```python
from build123d import *

# Parameters (mm, degrees)
SKETCH_1_W          = 109
SKETCH_1_H          = 31
SKETCH_1_W_2        = 9.6
SKETCH_1_H_2        = 9.7
SKETCH_1_H_3        = 5.6
SKETCH_1_W_3        = 14.8
SKETCH_1_H_4        = 16
SKETCH_1_W_4        = 9.5
SKETCH_1_H_5        = 3.5
SKETCH_1_W_5        = 15.5
SKETCH_1_H_6        = 6
SKETCH_1_W_6        = 80
SKETCH_1_H_7        = 8
EXTRUDE_1_DEPTH     = 2
SKETCH_2_W          = 2.5
SKETCH_2_H          = 8
EXTRUDE_2_DEPTH     = 2
SKETCH_3_W          = 15
SKETCH_3_H          = 2.5
EXTRUDE_4_DEPTH     = 2
CUT_EXTRUDE_2_DEPTH = 2


with BuildPart() as part:
    # 草图1 → 凸台-拉伸1 (new body)
    with BuildSketch(Plane.XY):
        with Locations((43, 12.2)):
            Rectangle(SKETCH_1_W, SKETCH_1_H)
        Polygon((27.2, 3.55), (32.1, 3.55), (32.1, 0.55), (39, 0.55), (39, 3.55), (43.9, 3.55), (43.9, 13.55), (27.2, 13.55), align=None, mode=Mode.SUBTRACT)
        with Locations((4.8, 4.85)):
            Rectangle(SKETCH_1_W_2, SKETCH_1_H_2, mode=Mode.SUBTRACT)
        with Locations((18.5, 6.9)):
            Rectangle(SKETCH_1_W_2, SKETCH_1_H_3, mode=Mode.SUBTRACT)
        with Locations((54.7, 6.55)):
            Rectangle(SKETCH_1_W_3, SKETCH_1_H_4, mode=Mode.SUBTRACT)
        with Locations((76.35, 12.8)):
            Rectangle(SKETCH_1_W_4, SKETCH_1_H_5, mode=Mode.SUBTRACT)
        with Locations((76.35, 3.55)):
            Rectangle(SKETCH_1_W_5, SKETCH_1_H_6, mode=Mode.SUBTRACT)
        with Locations((43, 20.2)):
            Rectangle(SKETCH_1_W_6, SKETCH_1_H_7, mode=Mode.SUBTRACT)
    extrude(amount=EXTRUDE_1_DEPTH)

    # 草图2 → 凸台-拉伸2 (add)
    with BuildSketch(Plane.XY.offset(2)):
        with Locations((-12.75, 18.7)):
            Rectangle(SKETCH_2_W, SKETCH_2_H)
        with Locations((-12.75, 5.7)):
            Rectangle(SKETCH_2_W, SKETCH_2_H)
        with Locations((98.75, 5.7)):
            Rectangle(SKETCH_2_W, SKETCH_2_H)
        with Locations((98.75, 18.7)):
            Rectangle(SKETCH_2_W, SKETCH_2_H)
    extrude(amount=-EXTRUDE_2_DEPTH)

    # 草图3 → 凸台-拉伸4 (add)
    with BuildSketch(Plane.XY):
        with Locations((6, 28.95)):
            Rectangle(SKETCH_3_W, SKETCH_3_H)
        with Locations((43, 28.95)):
            Rectangle(SKETCH_3_W, SKETCH_3_H)
        with Locations((80, 28.95)):
            Rectangle(SKETCH_3_W, SKETCH_3_H)
        with Locations((80, -4.55)):
            Rectangle(SKETCH_3_W, SKETCH_3_H)
        with Locations((43, -4.55)):
            Rectangle(SKETCH_3_W, SKETCH_3_H)
        with Locations((6, -4.55)):
            Rectangle(SKETCH_3_W, SKETCH_3_H)
    extrude(amount=EXTRUDE_4_DEPTH)

    # 草图4 → 切除-拉伸2 (cut)
    with BuildSketch(Plane.XY):
        with BuildLine():
            Line((-3.5, 27.7), (-1.5, 27.7))
            ThreePointArc((-1.5, 27.7), (-2.5, 26.7), (-3.5, 27.7))
        make_face()
        with BuildLine():
            Line((15.5, 27.7), (13.5, 27.7))
            ThreePointArc((13.5, 27.7), (14.5, 26.7), (15.5, 27.7))
        make_face()
        with BuildLine():
            Line((33.5, 27.7), (35.5, 27.7))
            ThreePointArc((35.5, 27.7), (34.5, 26.7), (33.5, 27.7))
        make_face()
        with BuildLine():
            Line((52.5, 27.7), (50.5, 27.7))
            ThreePointArc((50.5, 27.7), (51.5, 26.7), (52.5, 27.7))
        make_face()
        with BuildLine():
            Line((70.5, 27.7), (72.5, 27.7))
            ThreePointArc((72.5, 27.7), (71.5, 26.7), (70.5, 27.7))
        make_face()
        with BuildLine():
            Line((89.5, 27.7), (87.5, 27.7))
            ThreePointArc((87.5, 27.7), (88.5, 26.7), (89.5, 27.7))
        make_face()
        with BuildLine():
            Line((89.5, -3.3), (87.5, -3.3))
            ThreePointArc((87.5, -3.3), (88.5, -2.3), (89.5, -3.3))
        make_face()
        with BuildLine():
            Line((70.5, -3.3), (72.5, -3.3))
            ThreePointArc((72.5, -3.3), (71.5, -2.3), (70.5, -3.3))
        make_face()
        with BuildLine():
            Line((52.5, -3.3), (50.5, -3.3))
            ThreePointArc((50.5, -3.3), (51.5, -2.3), (52.5, -3.3))
        make_face()
        with BuildLine():
            Line((33.5, -3.3), (35.5, -3.3))
            ThreePointArc((35.5, -3.3), (34.5, -2.3), (33.5, -3.3))
        make_face()
        with BuildLine():
            Line((15.5, -3.3), (13.5, -3.3))
            ThreePointArc((13.5, -3.3), (14.5, -2.3), (15.5, -3.3))
        make_face()
        with BuildLine():
            Line((-3.5, -3.3), (-1.5, -3.3))
            ThreePointArc((-1.5, -3.3), (-2.5, -2.3), (-3.5, -3.3))
        make_face()
    extrude(amount=CUT_EXTRUDE_2_DEPTH, mode=Mode.SUBTRACT)


solid = part.part
```
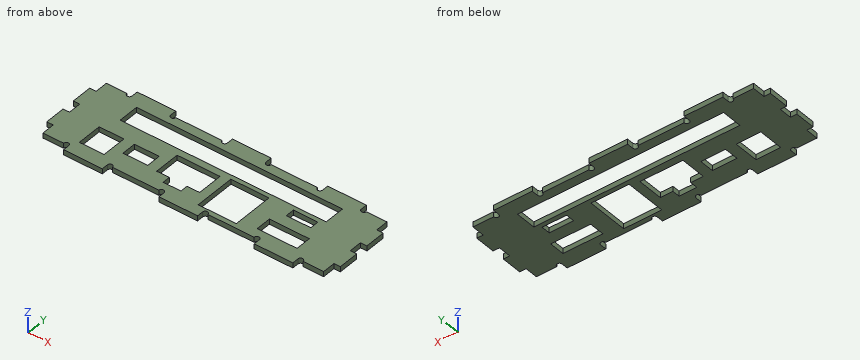
CAD build for the part. Positions are in the model's coordinates, mm. Round coordinates to 2 decimals unless told otherwise and drop trailing zeros. Write each loop counter-clockwise with the first axis right and the second up, starting at its lowest first coordinate (ties: lowest second). Pieces come first, ordered by that corner, then holes. Notation, with made-up numbers: (53, 48.25) - (90, 48.25) arc R23 cw to (90, 63.25) - close; hole circle Ø4 at (50.25, 52.25). An arc over 180 degrees is marked (long way). Write item = value, one per line. Start each with the question number.
Q1. Band-saw the part on A-A (x = 7). Give the cut face in (y, z), then the cut area to 3 significant figures.
Q2. Band-saw the part on B-B (y = 20). Give the cut face in (x, z), then the cut area to 3 significant figures.
Q3. Band-saw the part on D-D (z = 1.7). Count the separate pieces of the cut face and the enclosed holes in it, then the cut area to 3 significant figures.
Q4. Probe L1, parallel to Y at x = 81, z = 0.5; L2, parallel to Y at x = 8, z = 0.8; L3, parallel to X at y = 4, z = 0.5. List the from-to ranges inside material, lowest first. Write a range as from..to.
Q5. Band-saw the part on C-C (y = 8). Give the cut face in (x, z).
Q6. Drop flat-ended pins along their axis: pin 1 (0.6 mm diameter, centred on y = -1.5, z = 0.5, fed in from +X); pin 2 (0.6 mm diameter, centred on x = 25, z = 1, fed in from +Y). Give the stop position or say it passes through.
Answers below:
q1.outline = (-5.8, 0) - (0, 0) - (0, 2) - (-5.8, 2) - close; (9.7, 0) - (16.2, 0) - (16.2, 2) - (9.7, 2) - close; (24.2, 0) - (30.2, 0) - (30.2, 2) - (24.2, 2) - close
q1.area = 36.6 mm2
q2.outline = (-14, 0) - (3, 0) - (3, 2) - (-14, 2) - close; (83, 0) - (100, 0) - (100, 2) - (83, 2) - close
q2.area = 68.0 mm2
q3.separate_pieces = 1
q3.enclosed_holes = 7
q3.area = 2,330 mm2
q4.L1 = -5.8..0.55, 6.55..11.05, 14.55..16.2, 24.2..30.2
q4.L2 = -5.8..0, 9.7..16.2, 24.2..30.2
q4.L3 = -14..0, 9.6..27.2, 43.9..47.3, 62.1..68.6, 84.1..100
q5.outline = (-14, 0) - (0, 0) - (0, 2) - (-14, 2) - close; (9.6, 0) - (13.7, 0) - (13.7, 2) - (9.6, 2) - close; (23.3, 0) - (27.2, 0) - (27.2, 2) - (23.3, 2) - close; (43.9, 0) - (47.3, 0) - (47.3, 2) - (43.9, 2) - close; (62.1, 0) - (100, 0) - (100, 2) - (62.1, 2) - close
q6.pin_1 = 97.5
q6.pin_2 = 27.7
